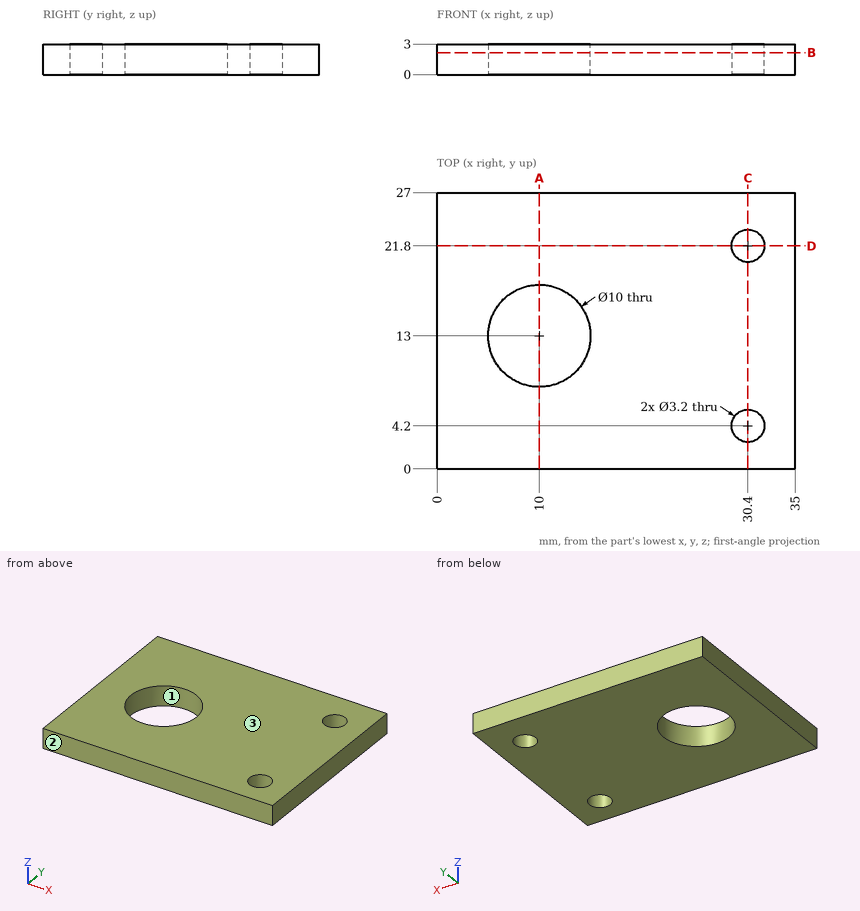
Input: dimensioned drawing with shaded views. Units: mm. Origin: part minimum x, y, z. Coordinates: 2 decimals unless noted, no trailing zeros. Order: outer loops, then holes, each group sorted by start corner. A loop starts at its lowest first (then second) coordinate and runs counter-clockwise, first axis right, second up. Notation, with made-up numbers: M -34.75,54 L 24.25,54 A30 cw 24.25,80 Z; hole C 75.25,-10 d7. An arc over 180 degrees is marked long. Write each question's results on one line, items separated by ' | '. Start each with the question number.
Item 1: Line query: probe 1 along Y at (x, z) = (30.4, 2.05); probe 2 along X at (y, z) = (4.2, 1.1); probe 3 along Y at (x, z) = (10, 2.3). Output: solid intervals per line, ascending.
Item 2: Cut plane C-C (x = 30.4). Return loops of the section in (y, z).
Item 3: Cut plane D-D (y = 21.8). Return loops of the section in (x, z), and give its area (3 significant figures).
Item 4: Draft query along Y for the marked faces 1, 2 and 3. Return one class per face: pulls with the +Y half, pulls with the -Y half, needs draft (parallel to the pull), parting line crosses it, or undercut.
Item 5: Cut plane B-B (z = 2.15). Return loops of the section in (x, y), and give its area (3 significant figures).
Item 6: Cut plane A-A (x = 10). Return loops of the section in (y, z), and give its area (3 significant figures).
Checked values:
1) probe 1: y = 0 to 2.6, 5.8 to 20.2, 23.4 to 27 | probe 2: x = 0 to 28.8, 32 to 35 | probe 3: y = 0 to 8, 18 to 27
2) outline: M 0,0 L 2.6,0 L 2.6,3 L 0,3 Z; M 5.8,0 L 20.2,0 L 20.2,3 L 5.8,3 Z; M 23.4,0 L 27,0 L 27,3 L 23.4,3 Z
3) outline: M 0,0 L 28.8,0 L 28.8,3 L 0,3 Z; M 32,0 L 35,0 L 35,3 L 32,3 Z | area: 95.4 mm2
4) face 1: undercut | face 2: pulls with the -Y half | face 3: needs draft
5) outline: M 0,0 L 35,0 L 35,27 L 0,27 Z; hole C 10,13 d10; hole C 30.4,4.2 d3.2; hole C 30.4,21.8 d3.2 | area: 850 mm2
6) outline: M 0,0 L 8,0 L 8,3 L 0,3 Z; M 18,0 L 27,0 L 27,3 L 18,3 Z | area: 51.0 mm2
